Geometry check sheet. Reference: the model listing, model coordinates, mm. A direction names the side the tool comes from. Round coordinates to 2 decimals unless told otherwise and drop trailing zeros. Write each loop counter-clockwise with the first axis right and the second up, starting at its lowest first coordinate (ties: lowest second). Pieces come first, ordered by that corner, then holes.
Item 1: Cross-section at C-C (y = -1.5). Enter the section's corners in (x, z).
Item 2: Depth check by flat-ended pin: P1, Ø1.5, axis at y = -19.5, z = -0.5, coming from the +X side; P2, Ø1.5, axis at x = -1, y = -42, coming from the -Z side. Enter the tip coordinate at first touch or a pass-through.
Item 3: Scan lines: probe 1 along Y at (x, z) = (0, 1.35); probe 2 along Y at (x, z) = (0.3, 0.1); probe 3 along X at (y, z) = (-1.5, -0.7). Record each from-to range of solid material in increasing order.
Item 4: Cross-section at D-D (y = -50). Enter the section's corners in (x, z), then the cut area to 3 significant figures.
Item 5: Cross-section at B-B (x = 0). Enter the section's corners in (y, z), then the cut area to 3 significant figures.
Item 6: Cross-section at A-A (z = 0). Enter the section's corners in (x, y), then the cut area to 3 significant figures.
Item 7: Access from +Z, -Z, +X, -X, +Y, -Y to the whole of each face (thin tool, end or side, straight path). Record for faces 4 (the face through (-1.5, -7.35, 0.07)), 5 (the face through (-0.97, -14.75, -1.27)).
Item 8: Draft check along X on faces 1 (the face through (-1.5, -37.82, 0.07)), 2 (the face through (0.28, -2.03, 1.26)), 3 (the face through (0, 0, 0)). Enter one of: pulls with the +X half, pulls with the -X half, needs draft (parallel to the pull), parting line crosses it, or undercut.
from build123d import *

# Parameters (mm, degrees)
SKETCH2_R           = 1.5
SKETCH4_R           = 0.5
CUT_EXTRUDE1_DEPTH  = 2
CUT_EXTRUDE2_START  = 1.6
SKETCH6_R           = 0.6
CUT_EXTRUDE2_DEPTH  = 0.5
BOSS_EXTRUDE1_START = -15
SKETCH7_R           = 1.6
BOSS_EXTRUDE1_DEPTH = 0.5


with BuildPart() as part:
    # Sweep1: sweep along a path in Sketch3
    with BuildLine(Plane(origin=(0, 0, 0), x_dir=(0, 0, -1), z_dir=(1, 0, 0))) as sweep1_path:
        Line((0, 0), (0, -60))
    # Sketch2 → Sweep1 (sweep)
    with BuildSketch(Plane(origin=(0, 0, 0), x_dir=(1, 0, 0), z_dir=(0, 1, 0))):
        Circle(SKETCH2_R)
    sweep(path=sweep1_path.line)

    # Sketch4 → Cut-Extrude1 (cut, symmetric)
    with BuildSketch(Plane.XY):
        with Locations(Location((0, -1.5, 0), (0, 0, 89.999999987))):
            Circle(SKETCH4_R)
    extrude(amount=CUT_EXTRUDE1_DEPTH, both=True, mode=Mode.SUBTRACT)

    # Sketch6 → Cut-Extrude2 (cut)
    with BuildSketch(Plane.XY.offset(CUT_EXTRUDE2_START)):
        with Locations((0, -1.5)):
            Circle(SKETCH6_R)
    extrude(amount=-CUT_EXTRUDE2_DEPTH, mode=Mode.SUBTRACT)

    # Sketch7 → Boss-Extrude1 (add)
    with BuildSketch(Plane(origin=(0, 0, 0), x_dir=(1, 0, 0), z_dir=(0, 1, 0)).offset(BOSS_EXTRUDE1_START)):
        with Locations(Location((0, 0, 0), (0, 0, 270))):
            Circle(SKETCH7_R)
    extrude(amount=BOSS_EXTRUDE1_DEPTH)


solid = part.part
Resolved:
1. outline: (-0.6, 1.1) - (-0.6, 1.37) arc R1.5 ccw to (-0.5, -1.41) - (-0.5, 1.1) - close; (0.5, -1.41) arc R1.5 ccw to (0.6, 1.37) - (0.6, 1.1) - (0.5, 1.1) - close
2. P1: stops at x = 1.5
2. P2: stops at z = -1.48
3. probe 1: y = -60 to -2.1, -0.9 to 0
3. probe 2: y = -60 to -1.9, -1.1 to 0
3. probe 3: x = -1.33 to -0.5, 0.5 to 1.33
4. outline: circle Ø3 at (0, 0)
4. area: 7.07 mm2
5. outline: (-60, -1.5) - (-15, -1.5) - (-15, -1.6) - (-14.5, -1.6) - (-14.5, -1.5) - (-2, -1.5) - (-2, 1.1) - (-2.1, 1.1) - (-2.1, 1.5) - (-14.5, 1.5) - (-14.5, 1.6) - (-15, 1.6) - (-15, 1.5) - (-60, 1.5) - close; (-1, -1.5) - (0, -1.5) - (0, 1.5) - (-0.9, 1.5) - (-0.9, 1.1) - (-1, 1.1) - close
5. area: 177 mm2
6. outline: (-1.6, -15) - (-1.5, -15) - (-1.5, -60) - (1.5, -60) - (1.5, -15) - (1.6, -15) - (1.6, -14.5) - (1.5, -14.5) - (1.5, 0) - (-1.5, 0) - (-1.5, -14.5) - (-1.6, -14.5) - close; hole circle Ø1 at (0, -1.5)
6. area: 179 mm2
7. face 4: +Y
7. face 5: +Y, -Y
8. face 1: parting line crosses it
8. face 2: undercut
8. face 3: needs draft
